Part model, mm, in its own coordinate system. A direction names the side the tool comes from. Give positions to 0.01 mm unless a question says otherwise; leave off trailing zeros. Order: outer loops, then holes, each group sorted by start corner. A loop starts at its lowest first (then second) coordinate and runs counter-clockwise, first axis right, second up. Notation, with made-up numbers: (67, 70) - (83, 70) arc R23 cw to (83, 82) - close; hole circle Ø6 at (53.5, 63.5). An arc over 180 degrees is marked (long way). One line per item, written item: value.
```python
from build123d import *

# Parameters (mm, degrees)
F0_W     = 482.6
F0_H     = 82.55
F1_DEPTH = 12.7
F2_R     = 3.175
F3_T     = -1.524
F4_W     = 14.1732
F4_H     = 82.55
F5_DEPTH = 25.4


with BuildPart() as f1:
    # F0 (on Top) → F1 (new body)
    with BuildSketch(Plane.XY):
        Rectangle(F0_W, F0_H)
    extrude(amount=-F1_DEPTH)

    # F2
    f2_edges = [f1.edges().sort_by_distance(p)[0] for p in [
        (0, -41.275, 0),
    ]]
    fillet(f2_edges, radius=F2_R)

    # F3
    f3_openings = [f1.faces().sort_by_distance(p)[0] for p in [
        (0, 0, -12.7),
        (241.3, 0.08388, -6.361664),
        (0, 41.275, -6.35),
        (-241.3, 0.08388, -6.361664),
    ]]
    offset(amount=F3_T, openings=f3_openings)

    # F4 (on face) → F5 (cut)
    with BuildSketch(Plane.XY):
        with Locations((-234.2134, 0)):
            Rectangle(F4_W, F4_H)
        with Locations((234.2134, 0)):
            Rectangle(F4_W, F4_H)
    extrude(amount=-F5_DEPTH, mode=Mode.SUBTRACT)


solid = f1.part
```
1) Which spindle directions (+Z, -Z, +X, -X, +Y, -Y) get a long thin tool onto all of the face, cutting with end or side? Do faces 1 (the face through (-3, 2, -1.524)), 2 (the face through (-3, -41.275, -8)). Say none if no direction does.
Answer:
face 1: -Z, +X, -X, +Y
face 2: +Z, -Z, +X, -X, -Y
2) Slice it at B-B on y = -19.5. Write the cut outline in (x, z), then the cut area to 3 significant figures.
Answer:
outline: (-227.13, -1.52) - (227.13, -1.52) - (227.13, 0) - (-227.13, 0) - close
area: 692 mm2
3) Wall check: line 1 along Y through (x, z) = (81.5, -3.5) (3 decimals); line 2 along Z through (x, y) = (-203.5, 25.5); line 3 along Y through (x, z) = (72, -0.5) (3 decimals). Give the ranges that are in metal, low to high. Write a range as [from, to].
Answer:
line 1: y = [-41.275, -39.751]
line 2: z = [-1.52, 0]
line 3: y = [-39.81, 41.275]
4) Slice it at A-A on x = 83.5. Write the cut outline in (y, z) (3 decimals).
Answer:
outline: (-41.275, -12.7) - (-39.751, -12.7) - (-39.751, -3.175) arc R1.651 cw to (-38.1, -1.524) - (41.275, -1.524) - (41.275, 0) - (-38.1, 0) arc R3.175 ccw to (-41.275, -3.175) - close
5) Drop flat-ended pins along their axis: P1, Ø3, axis at x = -71.5, z = -10, coming from the +Y side; P2, Ø6, axis at x = -54, y = -3, coming from the -Z side. Give the stop position or say it passes through.
Answer:
P1: stops at y = -39.75
P2: stops at z = -1.52
6) Slice it at C-C on z = -10.5. Write the cut outline in (x, y) (3 decimals).
Answer:
outline: (-227.127, -41.275) - (227.127, -41.275) - (227.127, -39.751) - (-227.127, -39.751) - close
